Work out the finished part from the listing and answer in its coordinate system (mm). A direction names the side the tool comes from. Coordinates: 2 decimals unless noted, no trailing zeros. Order: outer loops, then holes, each group sorted by start corner. A loop starts at its lowest first (then second) coordinate and runs counter-clockwise, first axis right, second up. Notation, with made-up numbers: (-34.5, 55) - (-25.5, 55) arc R17 cw to (-25.5, 69) - close; hole circle Ø1 at (-26.5, 18.25). An arc over 180 degrees is marked (long way). Answer as a JSON object with one key per item and string values. Group by question number.
1) A tool of negligible diameter and unlimited length cuts with its end or side. For faces 1 (the face through (-2.018, 15.368, 3.246)), 2 (the face through (-2.741, -12.345, 0.146)), from which of +Z, -Z, +X, -X, +Y, -Y can it reach the whole face along a straight path? Write none if from no direction.
2) Section A-A (x = 0) is taken. Give the vertices of the cut face in (y, z).
3) Section B-B (z = -0.5) is taken. Give the vertices of the cut face in (x, y).
4) Each of these flat-tipped pins is pushed along its axis until it touches: P1, Ø2, axis at y = 2.5, z = -2.5, coming from the -X side; P2, Ø4, axis at y = 7, z = -1, coming from the +X side; P3, Ø1, axis at y = -10.5, z = 2, coming from the +X side. Where does it stop, or does it pass through?
5) The mould has two halves that part along Y. Classify faces 3 (the face through (-2.75, -12.39, -0.19)), 4 (the face through (-0.534, 4.065, 0.049)), 5 (the face through (-3.2, -3.2, 3.5)): released by +Y, released by -Y, zero draft, split by the parting line, or undercut.
6) Find the intervals of material crossed by line 1 along Y through (x, z) = (-3, 1.5); line 2 along Y through (x, z) = (-1.5, 1.25); line 3 along Z through (x, y) = (2.5, 13), in increasing order.
7) Section C-C (z = 2.5) is taken. Give the vertices of the cut face in (x, y), plus the area to 3 significant figures.
from build123d import *


with BuildPart() as part:
    # Sketch → Revolution (revolve)
    with BuildSketch(Plane.XZ):
        Polygon((4.1, 3.5), (15.5, 3.5), (15.5, 3), (12.5, 0), (15.5, -3), (15.5, -3.5), (4.1, -3.5), align=None)
    revolve(axis=Axis((0, 0, 0), (0, 0, 1)))


solid = part.part
Report:
{
 "1": {"face 1": "+Z, -Z", "face 2": "none"},
 "2": {"outline": "(-15.5, -3.5) - (-4.1, -3.5) - (-4.1, 3.5) - (-15.5, 3.5) - (-15.5, 3) - (-12.5, 0) - (-15.5, -3) - close; (4.1, -3.5) - (15.5, -3.5) - (15.5, -3) - (12.5, 0) - (15.5, 3) - (15.5, 3.5) - (4.1, 3.5) - close"},
 "3": {"outline": "circle Ø26 at (0, 0); hole circle Ø8.2 at (0, 0)"},
 "4": {"P1": "stops at x = -15.41", "P2": "stops at x = 14.02", "P3": "stops at x = 10.86"},
 "5": {"face 3": "split by the parting line", "face 4": "undercut", "face 5": "zero draft"},
 "6": {"line 1": "y = -13.67 to -2.79, 2.79 to 13.67", "line 2": "y = -13.67 to -3.82, 3.82 to 13.67", "line 3": "z = -3.5 to -0.74, 0.74 to 3.5"},
 "7": {"outline": "circle Ø30 at (0, 0); hole circle Ø8.2 at (0, 0)", "area": "654 mm²"}
}
